Geometry check sheet. Reference: the model listing, model coordinates, mm. A direction names the side the tool comes from. Round coordinates to 2 decimals unless told otherwise and drop trailing zeros. Write each loop counter-clockwise with the first axis right and the second up, starting at its lowest first coordinate (ties: lowest second). Pieces come first, ordered by that corner, then holes.
Item 1: Draft check along Z on faces 1 (the face through (0, 0, 12.954)), 2 (the face through (3.785, 6.243, -108.888)), 3 (the face through (-0.517, -31.117, 1.628)). Enter one of: pulls with the +Z half, pulls with the -Z half, needs draft (parallel to the pull), parting line crosses it, or undercut.
Item 2: Access from +Z, -Z, +X, -X, +Y, -Y to the whole of each face (thin tool, end or side, straight path). Record for faces 4 (the face through (-1.72, -7.75, 8.06)), 5 (the face through (-44.067, 0.198, 1.628)), 6 (the face through (0, 0, -93.726)).
Item 3: Cross-section at C-C (z = -59). Enter the section's corners in (x, y) (1 decimal), then the cut area to 3 significant figures.
Item 4: Cross-section at B-B (y = 0). Enter the section's corners in (x, z).
Item 5: Scan lines: probe 1 along Y at (x, z) = (0, 2); probe 2 along Z at (x, y) = (1.5, 18); probe 3 along Y at (x, z) = (0.5, -10). Record each from-to range of solid material in increasing order.
Item 6: Depth check by flat-ended pin: P1, Ø4, axis at x = 4, z = -51, coming from the +Y side; P2, Ø13, axis at x = -2.5, y = 2, coming from the -Z side; P3, Ø12, axis at y = 7.5, z = -104.5, coming from the +X side; P4, Ø8, axis at y = -9.5, z = -35.5, coming from the -X side. Enter the tip coordinate at first touch or a pass-through.
Item 7: Cross-section at A-A (x = 0). Enter the section's corners in (y, z), then the cut area to 3 significant figures.
from build123d import *

# Parameters (mm, degrees)
SKETCH1_R           = 3.96875
BOSS_EXTRUDE1_DEPTH = 3.302
SKETCH2_R           = 7.9375
BOSS_EXTRUDE2_DEPTH = 9.652
SKETCH3_R           = 7.9375
BOSS_EXTRUDE3_DEPTH = 119.126
SKETCH4_R           = 6
CUT_EXTRUDE1_DEPTH  = 25.4
CUT_EXTRUDE2_REACH  = 56.229
SKETCH5_R           = 3.96875


with BuildPart() as part:
    # Sketch1 → Boss-Extrude1 (new body)
    with BuildSketch(Plane.XY):
        with BuildLine():
            ThreePointArc((9.017, 35.052), (0, 44.069), (-9.017, 35.052))
            add(Edge.make_bspline(
                [(-9.017, 35.052), (-13.886524484, 13.886524484), (-35.052, 9.017)],
                knots=[0, 0, 0, 1, 1, 1], degree=2))
            ThreePointArc((-35.052, 9.017), (-44.069, 0), (-35.052, -9.017))
            add(Edge.make_bspline(
                [(-35.052, -9.017), (-13.886524484, -13.886524484), (-9.017, -35.052)],
                knots=[0, 0, 0, 1, 1, 1], degree=2))
            ThreePointArc((-9.017, -35.052), (0, -44.069), (9.017, -35.052))
            add(Edge.make_bspline(
                [(35.052, -9.017), (13.886524484, -13.886524484), (9.017, -35.052)],
                knots=[0, 0, 0, 1, 1, 1], degree=2))
            ThreePointArc((35.052, -9.017), (44.069, 0), (35.052, 9.017))
            add(Edge.make_bspline(
                [(9.017, 35.052), (13.886524484, 13.886524484), (35.052, 9.017)],
                knots=[0, 0, 0, 1, 1, 1], degree=2))
        make_face()
        with Locations((0, 35.052)):
            Circle(SKETCH1_R, mode=Mode.SUBTRACT)
        with Locations((35.052, 0)):
            Circle(SKETCH1_R, mode=Mode.SUBTRACT)
        with Locations((0, -35.052)):
            Circle(SKETCH1_R, mode=Mode.SUBTRACT)
        with Locations((-35.052, 0)):
            Circle(SKETCH1_R, mode=Mode.SUBTRACT)
    extrude(amount=BOSS_EXTRUDE1_DEPTH)

    # Sketch2 → Boss-Extrude2 (add)
    with BuildSketch(Plane.XY.offset(3.302)):
        Circle(SKETCH2_R)
    extrude(amount=BOSS_EXTRUDE2_DEPTH)

    # Sketch3 → Boss-Extrude3 (add)
    with BuildSketch(Plane(origin=(0, 0, 0), x_dir=(-1, 0, 0), z_dir=(0, 0, -1))):
        Circle(SKETCH3_R)
    extrude(amount=BOSS_EXTRUDE3_DEPTH)

    # Sketch4 → Cut-Extrude1 (cut)
    with BuildSketch(Plane(origin=(0, 0, -119.126), x_dir=(-1, 0, 0), z_dir=(0, 0, -1))):
        Circle(SKETCH4_R)
    extrude(amount=-CUT_EXTRUDE1_DEPTH, mode=Mode.SUBTRACT)

    # Sketch5 → Cut-Extrude2 (cut, up to next)
    with BuildSketch(Plane(origin=(0, 10.16, 0), x_dir=(1, 0, 0), z_dir=(0, 1, 0)), mode=Mode.PRIVATE) as cut_extrude2_sk1:
        with Locations((0, 107.696)):
            Circle(SKETCH5_R)
    cut_extrude2_tool1 = extrude(cut_extrude2_sk1.sketch, amount=-CUT_EXTRUDE2_REACH, mode=Mode.PRIVATE) & part.part
    add(cut_extrude2_tool1.solids().sort_by_distance((0, 10.16, -107.696))[0], mode=Mode.SUBTRACT)


solid = part.part
Resolved:
1. face 1: pulls with the +Z half
1. face 2: undercut
1. face 3: needs draft
2. face 4: +Z
2. face 5: +Z, -Z, -X
2. face 6: -Z
3. outline: circle Ø15.9 at (0, 0)
3. area: 198 mm2
4. outline: (-44.07, 0) - (-39.02, 0) - (-39.02, 3.3) - (-44.07, 3.3) - close; (-31.08, 0) - (-7.94, 0) - (-7.94, -119.13) - (-6, -119.13) - (-6, -93.73) - (6, -93.73) - (6, -119.13) - (7.94, -119.13) - (7.94, 0) - (31.08, 0) - (31.08, 3.3) - (7.94, 3.3) - (7.94, 12.95) - (-7.94, 12.95) - (-7.94, 3.3) - (-31.08, 3.3) - close; (39.02, 0) - (44.07, 0) - (44.07, 3.3) - (39.02, 3.3) - close
5. probe 1: y = -44.07 to -39.02, -31.08 to 31.08, 39.02 to 44.07
5. probe 2: z = 0 to 3.3
5. probe 3: y = -7.92 to 7.92
6. P1: stops at y = 7.68
6. P2: stops at z = -119.13
6. P3: stops at x = 7.79
6. P4: stops at x = -5.72
7. outline: (-44.07, 0) - (-39.02, 0) - (-39.02, 3.3) - (-44.07, 3.3) - close; (-31.08, 0) - (-7.94, 0) - (-7.94, -119.13) - (-6, -119.13) - (-6, -93.73) - (6, -93.73) - (6, -103.73) - (7.94, -103.73) - (7.94, 0) - (31.08, 0) - (31.08, 3.3) - (7.94, 3.3) - (7.94, 12.95) - (-7.94, 12.95) - (-7.94, 3.3) - (-31.08, 3.3) - close; (6, -119.13) - (7.94, -119.13) - (7.94, -111.66) - (6, -111.66) - close; (39.02, 0) - (44.07, 0) - (44.07, 3.3) - (39.02, 3.3) - close
7. area: 1,960 mm2
